from build123d import *

# Parameters (mm, degrees)
SKETCH1_W           = 5.0165
SKETCH1_H           = 1.27
SKETCH2_W           = 6.2992
SKETCH2_H           = 6.2992
BOSS_EXTRUDE1_DEPTH = 3.81
SKETCH3_W           = 3.175
SKETCH3_H           = 3.175
CUT_EXTRUDE1_DEPTH  = 6.08
FILLET1_R           = 0.635
FILLET2_R           = 0.254
FILLET3_R           = 0.508
SKETCH4_R           = 1.7018
CUT_EXTRUDE2_DEPTH  = 51.054


with BuildPart() as part:
    # Sketch1 → Revolve1 (revolve)
    with BuildSketch(Plane.XY):
        with Locations((2.50825, 0.635)):
            Rectangle(SKETCH1_W, SKETCH1_H)
    revolve(axis=Axis((0, 1.27, 0), (0, -1, 0)))

    # Sketch2 → Boss-Extrude1 (add)
    with BuildSketch(Plane(origin=(0, 1.27, 0), x_dir=(-1, 0, 0), z_dir=(0, 1, 0))):
        Rectangle(SKETCH2_W, SKETCH2_H)
    extrude(amount=BOSS_EXTRUDE1_DEPTH)

    # Sketch3 → Cut-Extrude1 (cut, through all)
    with BuildSketch(Plane.XZ):
        Rectangle(SKETCH3_W, SKETCH3_H)
    extrude(amount=-CUT_EXTRUDE1_DEPTH, mode=Mode.SUBTRACT)

    # Fillet1
    fillet1_edges = [part.edges().sort_by_distance(p)[0] for p in [
        (3.1496, 3.175, 3.1496),
        (3.1496, 3.175, -3.1496),
        (-3.1496, 3.175, -3.1496),
        (-3.1496, 3.175, 3.1496),
    ]]
    fillet(fillet1_edges, radius=FILLET1_R)

    # Fillet2
    fillet2_edges = [part.edges().sort_by_distance(p)[0] for p in [
        (-1.5875, 2.54, -1.5875),
        (-1.5875, 2.54, 1.5875),
        (1.5875, 2.54, 1.5875),
        (1.5875, 2.54, -1.5875),
    ]]
    fillet(fillet2_edges, radius=FILLET2_R)

    # Fillet3
    fillet3_edges = [part.edges().sort_by_distance(p)[0] for p in [
        (0, 5.08, 3.1496),
        (-3.1496, 5.08, 0),
        (3.1496, 5.08, 0),
        (0, 5.08, -3.1496),
        (2.963612806, 5.08, -2.963612806),
        (-2.963612806, 5.08, -2.963612806),
        (2.963612806, 5.08, 2.963612806),
        (-2.963612806, 5.08, 2.963612806),
    ]]
    fillet(fillet3_edges, radius=FILLET3_R)

    # Sketch4 → Cut-Extrude2 (cut)
    with BuildSketch(Plane(origin=(0, 5.08, 0), x_dir=(1, 0, 0), z_dir=(0, 1, 0))):
        Circle(SKETCH4_R)
    extrude(amount=-CUT_EXTRUDE2_DEPTH, mode=Mode.SUBTRACT)


solid = part.part
Model file for the job. Use its own axes, mm. A direction names the side the tool comes from. Give positions to 0.01 mm unless a question says otherwise; leave off trailing zeros. Loops run counter-clockwise (first coordinate to the right, second up) from the corner with the lowest first, then second, coordinate; pieces in that order, holes last.
1) Saw through at D-D (x = 2). Write the cut outline in (y, z).
2) Wall check: line 1 (Z direction, x = -1, y = 4.5); line 2 (X direction, y = 2.9, z = 0); line 3 (Z direction, x = -2.5, y = 2.6). Give the ranges that are in metal, low to high.
3) Pull direction Z, two halves, no side cores. Call faces 1 (the flat face through (0, 3, -3.15)), 2 (the cylindrical face through (0, 2.6, 1.7)), 3 (the flat face through (2, 5.08, 0)): +Z half, -Z half, draft (parallel to the pull), parting line (faces both ways), or undercut.
4) Saw through at C-C (x = 0). Write the cut outline in (y, z), plus the area to 3 significant figures.
5) Flat gauge pins, fed straight in: pin 1 Ø2 at (y, z) = (3.5, 0.5) entering from -X; pin 2 Ø0.8 at (y, z) = (1.5, -1) entering from +X; pin 3 Ø0.6 at (y, z) = (2.5, 1) entering from +X. Where does each tip first touch, or does it go through?
6) Saw through at A-A (z = 0). Write the cut outline in (x, y).
7) Tool access for faces 4 (the cylindrical face through (1.7, 2.6, 0)), 5 (the flat face through (0, 3, 3.15)), 6 (the flat face through (-3.15, 3, 0)), 7 (the flat face through (3.15, 3, 0)): list every direction of +Z, -Z, +X, -X, +Y, -Y with a clear straight run to the whole face (end or side of a thin tool).
Answer block:
1. outline: (0, -4.6) - (1.27, -4.6) - (1.27, -3.15) - (4.57, -3.15) arc R0.51 ccw to (5.08, -2.64) - (5.08, 2.64) arc R0.51 ccw to (4.57, 3.15) - (1.27, 3.15) - (1.27, 4.6) - (0, 4.6) - close
2. line 1: z = -3.15 to -1.59, 1.59 to 3.15
2. line 2: x = -3.15 to -1.7, 1.7 to 3.15
2. line 3: z = -3.15 to 3.15
3. face 1: -Z half
3. face 2: undercut
3. face 3: draft
4. outline: (0, -5.02) - (1.27, -5.02) - (1.27, -3.15) - (4.57, -3.15) arc R0.51 ccw to (5.08, -2.64) - (5.08, -1.7) - (0, -1.7) - close; (0, 1.7) - (5.08, 1.7) - (5.08, 2.64) arc R0.51 ccw to (4.57, 3.15) - (1.27, 3.15) - (1.27, 5.02) - (0, 5.02) - close
4. area: 19.3 mm2
5. pin 1: stops at x = -3.15
5. pin 2: stops at x = 4.97
5. pin 3: stops at x = 3.15
6. outline: (-5.02, 0) - (-1.7, 0) - (-1.7, 5.08) - (-2.64, 5.08) arc R0.51 ccw to (-3.15, 4.57) - (-3.15, 1.27) - (-5.02, 1.27) - close; (1.7, 0) - (5.02, 0) - (5.02, 1.27) - (3.15, 1.27) - (3.15, 4.57) arc R0.51 ccw to (2.64, 5.08) - (1.7, 5.08) - close
7. face 4: +Y, -Y
7. face 5: +Z, +X, -X, +Y
7. face 6: +Z, -Z, -X, +Y
7. face 7: +Z, -Z, +X, +Y
